```python
from build123d import *

# Parameters (mm, degrees)
F0_W           = 53.4372702241
F0_H           = 47.1505336463
F1_DEPTH       = 181.102
F3_D           = 6.7564
F3_DEPTH       = 12.7
F3_CSINK_D     = 13.4874
F3_CSINK_ANGLE = 82
F3_TIP         = 2.0298273432


with BuildPart() as f1:
    # F0 (on Front) → F1 (new body)
    with BuildSketch(Plane.XZ):
        with Locations((26.718635112, 23.5752668232)):
            Rectangle(F0_W, F0_H)
    extrude(amount=-F1_DEPTH)

    # F3
    with Locations(Plane.XY.offset(47.1505336463)):
        with Locations((26.718635112, 137.7135068178)):
            CounterSinkHole(F3_D / 2, F3_CSINK_D / 2, depth=F3_DEPTH, counter_sink_angle=F3_CSINK_ANGLE)
            with Locations((0, 0, -(F3_DEPTH + F3_TIP / 2))):  # 118° drill point
                Cone(0, F3_D / 2, F3_TIP, mode=Mode.SUBTRACT)


solid = f1.part
```
Geometry: final body of the model. Coordinates: model frame, mm. A direction names the side the tool comes from. Coordinates: 2 decimals unless noted, no trailing zeros. Answer as CSV lines item,"result". Start each with the question number.
Q1. Line query: line 1 (Y direction, x = 24, z = 39.5). Output: solid intervals per line, ascending. Write a range as from..to.
Q2. Reachability of faces 4 (the flat face through (26, 89, 0)), 5 (the cylindrical face through (27.158, 141.063, 38.803)) from +Z, -Z, +X, -X, +Y, -Y: full face, straight path, thin tool, end or side. Return the list, or none.
Q3. Mould query, pull axis Y, two halves, no side actions, for faces 1 (the conical face through (27.261, 137.489, 32.773)), 2 (the flat face through (26, 181.102, 24)), 3 (the flat face through (53.437, 89, 23)). Classes: released by +Y, released by -Y, zero draft, split by the parting line, or undercut.
Q4. Pin query (flat end, axial travel): P1, Ø5.5, axis at x = 26.72, y = 137.71, coming from the +Z side. Return the tip coordinate at first contact, or that it passes through.
Findings below:
1,line 1,"y = 0..135.71, 139.72..181.1"
2,face 4,"-Z, +X, -X, +Y, -Y"
2,face 5,"+Z"
3,face 1,"undercut"
3,face 2,"released by +Y"
3,face 3,"zero draft"
4,P1,"stops at z = 34.08"
